from build123d import *

# Parameters (mm, degrees)
SKETCH_1_R          = 21
EXTRUDE_1_DEPTH     = 6
SKETCH_3_R          = 10
CUT_EXTRUDE_1_DEPTH = 13
SKETCH_2_R          = 17.75
SKETCH_2_R_2        = 13.3
CUT_EXTRUDE_2_DEPTH = 0.5


with BuildPart() as part:
    # 草圖1 → 填料-伸長1 (new body, symmetric)
    with BuildSketch(Plane.XY):
        Circle(SKETCH_1_R)
    extrude(amount=EXTRUDE_1_DEPTH, both=True)

    # 草圖3 → 除料-伸長1 (cut, through all)
    with BuildSketch(Plane.XY.offset(6)):
        Circle(SKETCH_3_R)
    extrude(amount=-CUT_EXTRUDE_1_DEPTH, mode=Mode.SUBTRACT)

    # 草圖2 → 除料-伸長2 (cut)
    with BuildSketch(Plane.XY.offset(6)):
        Circle(SKETCH_2_R)
        Circle(SKETCH_2_R_2, mode=Mode.SUBTRACT)
    cut_extrude_2 = extrude(amount=-CUT_EXTRUDE_2_DEPTH, mode=Mode.SUBTRACT)

    # 鏡射1: 除料-伸長2 across plane
    add(cut_extrude_2.mirror(Plane.XY), mode=Mode.SUBTRACT)


solid = part.part
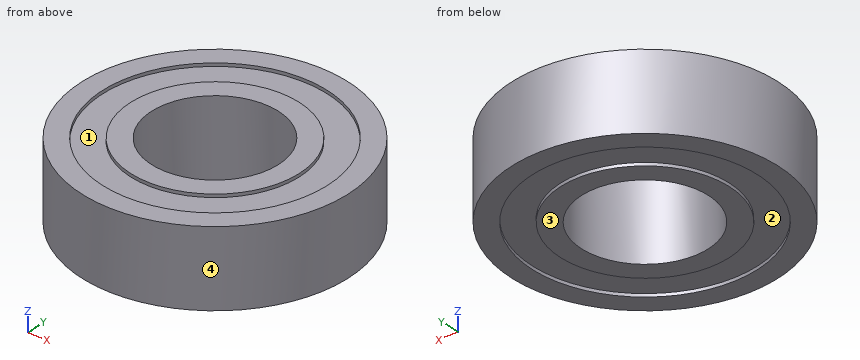
Source: CAD feature listing. Evaluate the final solid. Frame: model axes, mm. Face numbers are marked on the shaded views. Give positions to 0.01 mm unless a question says otherwise; leave off trailing zeros. Loops run counter-clockwise (first coordinate to the right, second up) from the corner with the lowest first, then second, coordinate; pieces in that order, holes last. Notation, with made-up numbers: (71.5, -14) -> (88.5, -14) arc R23 cw to (88.5, 10) -> close; hole circle Ø1 at (80, 87). An arc over 180 degrees is marked (long way). Use a Markdown table: item, result. Add a question column.
1) Pull-direction query (Y, two-part tool) for the marked faces 1, 2, 3 and 4; classes: +Y half, -Y half, draft (parallel to the pull), parting line (faces both ways), or undercut.
2) Section query A-A, the plane y = 0. Return the cut outline in (x, z).
3) Section query D-D, the plane z = 4.75. Return the cut outline in (x, y), then the cut area to 3 significant figures.
4) First-contact query: pin 1 (4 mm diameter, centred on x = 8, z = 0.5, fed in from +Y); pin 2 (4 mm diameter, centred on x = -14, z = -2.5, fed in from +Y); pin 3 (4 mm diameter, centred on x = -12, z = -4.5, fed in from +Y). Flat tips, straight axial feed; report the tip coordinate or a pass-through.
5) Line query: line 1 along Y through (x, z) = (0, 5.7); line 2 along Y through (x, z) = (0, 1.5); line 3 along Z through (x, y) = (-6, 15.5). Output: solid intervals per line, ascending. Write a range as [from, to].
6) Section query C-C, the plane y = 12. Return the cut outline in (x, z), then the cut area to 3 significant figures.
Numbers:
| question | item | result |
|---|---|---|
| 1 | face 1 | undercut |
| 1 | face 2 | undercut |
| 1 | face 3 | draft |
| 1 | face 4 | parting line |
| 2 | outline | (-21, -6) -> (-17.75, -6) -> (-17.75, -5.5) -> (-13.3, -5.5) -> (-13.3, -6) -> (-10, -6) -> (-10, 6) -> (-13.3, 6) -> (-13.3, 5.5) -> (-17.75, 5.5) -> (-17.75, 6) -> (-21, 6) -> close; (10, -6) -> (13.3, -6) -> (13.3, -5.5) -> (17.75, -5.5) -> (17.75, -6) -> (21, -6) -> (21, 6) -> (17.75, 6) -> (17.75, 5.5) -> (13.3, 5.5) -> (13.3, 6) -> (10, 6) -> close |
| 3 | outline | circle Ø42 at (0, 0); hole circle Ø20 at (0, 0) |
| 3 | area | 1,070 mm2 |
| 4 | pin 1 | stops at y = 20.12 |
| 4 | pin 2 | stops at y = 17.23 |
| 4 | pin 3 | stops at y = 18.47 |
| 5 | line 1 | y = [-21, -17.75], [-13.3, -10], [10, 13.3], [17.75, 21] |
| 5 | line 2 | y = [-21, -10], [10, 21] |
| 5 | line 3 | z = [-5.5, 5.5] |
| 6 | outline | (-17.23, -6) -> (-13.08, -6) -> (-13.08, -5.5) -> (-5.73, -5.5) -> (-5.73, -6) -> (5.73, -6) -> (5.73, -5.5) -> (13.08, -5.5) -> (13.08, -6) -> (17.23, -6) -> (17.23, 6) -> (13.08, 6) -> (13.08, 5.5) -> (5.73, 5.5) -> (5.73, 6) -> (-5.73, 6) -> (-5.73, 5.5) -> (-13.08, 5.5) -> (-13.08, 6) -> (-17.23, 6) -> close |
| 6 | area | 399 mm2 |
